Verification items for the finished model (mm, model axes). Face numbers are marked on the shaded views. A direction names the side the tool comes from. Give positions to 0.01 mm unless a question says otherwise; leave off trailing zeros. Write each loop counter-clockwise with the first axis right and the second up, starting at its lowest first coordinate (ties: lowest second). Pieces come first, ordered by that corner, then holes.
from build123d import *

# Parameters (mm, degrees)
F1_DEPTH = 25.4
F2_W     = 38.1
F2_H     = 12.7
F3_DEPTH = 19.05
F5_DEPTH = 25.4
F7_DEPTH = 25.4


with BuildPart() as f1:
    # F0 (on Front) → F1 (new body)
    with BuildSketch(Plane.XZ):
        Polygon((19.05, 0), (0, 0), (-19.05, 0), (-19.05, -31.75), (19.05, -31.75), align=None)
    extrude(amount=F1_DEPTH)

    # F2 (on face) → F3 (cut)
    with BuildSketch(Plane.XY):
        with Locations((0, -19.05)):
            Rectangle(F2_W, F2_H)
    extrude(amount=-F3_DEPTH, mode=Mode.SUBTRACT)

    # F4 (on face) → F5 (cut)
    with BuildSketch(Plane.XY.offset(-19.05)):
        Polygon((19.05, -25.4), (19.05, -12.7), (4.850968, -25.4), align=None)
    extrude(amount=-F5_DEPTH, mode=Mode.SUBTRACT)

    # F6 (on face) → F7 (cut)
    with BuildSketch(Plane.XZ.offset(12.7)):
        Polygon((19.05, -19.05), (19.05, 0), (6.35, 0), align=None)
    extrude(amount=-F7_DEPTH, mode=Mode.SUBTRACT)


solid = f1.part
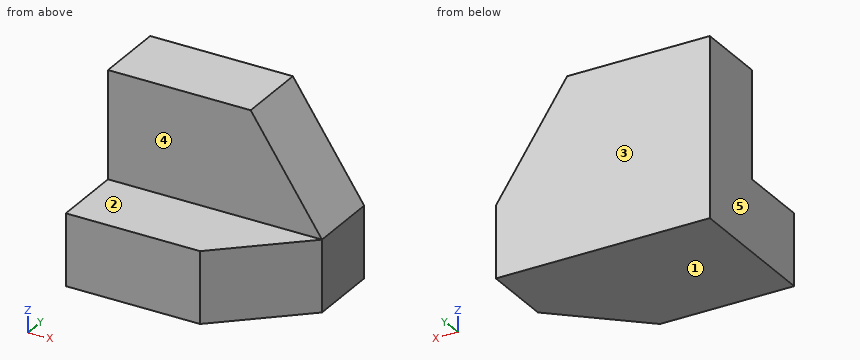
Item 1: Release check for a two-part mould opening along Z. For the marked faces 1, 2 and 3 record: released by +Z, released by -Z, zero draft, split by the parting line, or undercut.
Answer key:
face 1: released by -Z
face 2: released by +Z
face 3: zero draft
Item 2: Set-up check for the marked faces 4 and 5: record each of +Z, -Z, +X, -X, +Y, -Y from which the full face is reachable in a straight line by a thin tool's end or side.
Answer key:
face 4: +Z, +X, -X, -Y
face 5: +Z, -Z, -X, +Y, -Y
Item 3: Depth check by flat-ended pin: pin 1 (5 mm diameter, centred on x = 6.5, y = -5, fed in from +Z); pin 2 (4 mm diameter, centred on x = 1, y = -19, fed in from +Z); pin 3 (8 mm diameter, centred on y = -5.5, z = -15, fed in from +X); pin 4 (8 mm diameter, centred on y = -23, z = -15, fed in from +X). Enter the tip coordinate at first touch or a pass-through.
Answer key:
pin 1: stops at z = 0
pin 2: stops at z = -19.05
pin 3: stops at x = 19.02
pin 4: passes through
Item 4: Sectioned sample at C-C on y = -5.75. Record the cut outline in (x, z).
Answer key:
outline: (-19.05, -31.75) - (19.05, -31.75) - (19.05, -19.05) - (6.35, 0) - (-19.05, 0) - close
Item 5: Sectioned sample at B-B on x = -3.5. Record the cut outline in (y, z), then the cut area to 3 significant figures.
Answer key:
outline: (-25.4, -31.75) - (0, -31.75) - (0, 0) - (-12.7, 0) - (-12.7, -19.05) - (-25.4, -19.05) - close
area: 565 mm2
Item 6: Sectioned sample at D-D on z = -7.5. Record the cut outline in (x, y), then the cut area to 3 significant figures.
Answer key:
outline: (-19.05, -12.7) - (11.35, -12.7) - (11.35, 0) - (-19.05, 0) - close
area: 386 mm2
Item 7: Sectioned sample at A-A on z = -23. Record the cut outline in (x, y).
Answer key:
outline: (-19.05, -25.4) - (4.85, -25.4) - (19.05, -12.7) - (19.05, 0) - (-19.05, 0) - close
Item 8: Scan lines: line 1 along Z through (x, y) = (-12.5, -23.5); line 2 along Y through (x, z) = (-16, -12); line 3 along Y through (x, z) = (15, -22). Record each from-to range of solid material in increasing order.
Answer key:
line 1: z = -31.75 to -19.05
line 2: y = -12.7 to 0
line 3: y = -16.32 to 0
